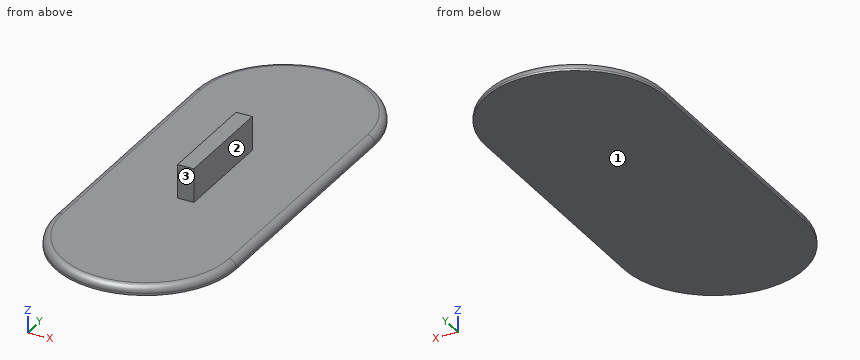
from build123d import *

# Parameters (mm, degrees)
F2_DEPTH = 1
F4_DEPTH = 2
F5_W     = 1.8
F5_H     = 11.8
F6_DEPTH = 7.5
F7_R     = 1.5


with BuildPart() as f2:
    # F1 (on Top) → F2 (new body)
    with BuildSketch(Plane.XY):
        with BuildLine():
            Line((0, 23), (0, 0))
            Line((0, 0), (-5, 0))
            Line((-5, 0), (-5, -28))
            ThreePointArc((-5, -28), (0, -23), (5, -28))
            Line((5, -28), (5, 0))
            Line((5, 0), (5, 28))
            ThreePointArc((5, 28), (3.5355339059, 24.4644660941), (0, 23))
        make_face()
        with BuildLine():
            Line((-5, 0), (0, 0))
            Line((0, 0), (0, 23))
            ThreePointArc((0, 23), (-3.5355339059, 24.4644660941), (-5, 28))
            Line((-5, 28), (-5, 0))
        make_face()
        with BuildLine():
            ThreePointArc((-5, 28), (-3.5355339059, 24.4644660941), (0, 23))
            Line((0, 23), (0, 28))
            Line((0, 28), (-5, 28))
        make_face()
        with BuildLine():
            Line((0, 28), (0, 23))
            ThreePointArc((0, 23), (3.5355339059, 24.4644660941), (5, 28))
            Line((5, 28), (0, 28))
        make_face()
        with BuildLine():
            ThreePointArc((5, 28), (0, 33), (-5, 28))
            Line((-5, 28), (0, 28))
            Line((0, 28), (5, 28))
        make_face()
        with BuildLine():
            ThreePointArc((5, -28), (0, -23), (-5, -28))
            ThreePointArc((-5, -28), (0, -33), (5, -28))
        make_face()
    extrude(amount=F2_DEPTH)

    # F3 (on Top) → F4 (join)
    with BuildSketch(Plane.XY):
        with BuildLine():
            Line((-20, 28), (-20, -28))
            ThreePointArc((-20, -28), (0, -48), (20, -28))
            Line((20, -28), (20, 28))
            ThreePointArc((20, 28), (0, 48), (-20, 28))
        make_face()
    extrude(amount=F4_DEPTH)

    # F5 (on face) → F6 (join)
    with BuildSketch(Plane.XY.offset(2)):
        with Locations((-0.9, -5.9)):
            Rectangle(F5_W, F5_H)
        with Locations((-0.9, 5.9)):
            Rectangle(F5_W, F5_H)
        with Locations((0.9, 5.9)):
            Rectangle(F5_W, F5_H)
        with Locations((0.9, -5.9)):
            Rectangle(F5_W, F5_H)
    extrude(amount=F6_DEPTH)

    # F7
    f7_edges = [f2.edges().sort_by_distance(p)[0] for p in [
        (-20, 0, 2),
    ]]
    fillet(f7_edges, radius=F7_R)


solid = f2.part
CAD build for the part. Positions are in the model's coordinates, mm. Face numbers are marked on the shaded views. A direction names the side the tool comes from. Round coordinates to 2 decimals unless told otherwise and drop trailing zeros. Loops run counter-clockwise (first coordinate to the right, second up) from the corner with the lowest first, then second, coordinate; pieces in that order, holes last.
(1) Wall check: line 1 along Z through (x, y) = (-7, -43.5); line 2 along X through (y, z) = (0, 2.25); line 3 along Y through (x, z) = (-1, 2.75). Give the ranges that are in metal, low to high.
(2) Which spindle directions (+Z, -Z, +X, -X, +Y, -Y) get a long thin tool onto all of the face, cutting with end or side? Do the marked faces 1, 2 and 3. Say none if no direction does.
(3) Drop flat-ended pins along their axis: pin 1 (4 mm diameter, centred on y = 2, z = 7.5, fed in from -X); pin 2 (2 mm diameter, centred on x = 0.5, z = 4, fed in from -Y); pin 3 (1.1 mm diameter, centred on x = -0.5, z = 5.5, fed in from +Y). Give the stop position or say it passes through.
(4) Cut at B-B (x = 0). Give the cut face in (y, z), plus the area to 3 significant figures.
(5) Cut at A-A (y = 6). Give the cut face in (x, z).
(6) Cut at C-C (z = 3). Give the cut face in (x, y).
(7) Cut at D-D (y = 23.5). Give the cut face in (x, z).
Findings below:
1. line 1: z = 0 to 2
1. line 2: x = -1.8 to 1.8
1. line 3: y = -11.8 to 11.8
2. face 1: -Z, +X, -X, +Y, -Y
2. face 2: +Z, +X, +Y, -Y
2. face 3: +Z, +X, -X, -Y
3. pin 1: stops at x = -1.8
3. pin 2: stops at y = -11.8
3. pin 3: stops at y = 11.8
4. outline: (-48, 0) - (48, 0) - (48, 0.5) arc R1.5 ccw to (46.5, 2) - (11.8, 2) - (11.8, 9.5) - (-11.8, 9.5) - (-11.8, 2) - (-46.5, 2) arc R1.5 ccw to (-48, 0.5) - close
4. area: 368 mm2
5. outline: (-20, 0) - (20, 0) - (20, 0.5) arc R1.5 ccw to (18.5, 2) - (1.8, 2) - (1.8, 9.5) - (-1.8, 9.5) - (-1.8, 2) - (-18.5, 2) arc R1.5 ccw to (-20, 0.5) - close
6. outline: (-1.8, -11.8) - (1.8, -11.8) - (1.8, 11.8) - (-1.8, 11.8) - close
7. outline: (-20, 0) - (20, 0) - (20, 0.5) arc R1.5 ccw to (18.5, 2) - (-18.5, 2) arc R1.5 ccw to (-20, 0.5) - close
